Part print with two shaded views. Sizes in mm from the minimum x, y, z corner. A direction names the side the tool comes from. Coordinates: 2 decimals unless noted, no trailing zeros. Order: outer loops, then holes, each group sorted by start corner. A loop starts at its lowest first (then second) coordinate and runs counter-clockwise, first axis right, second up.
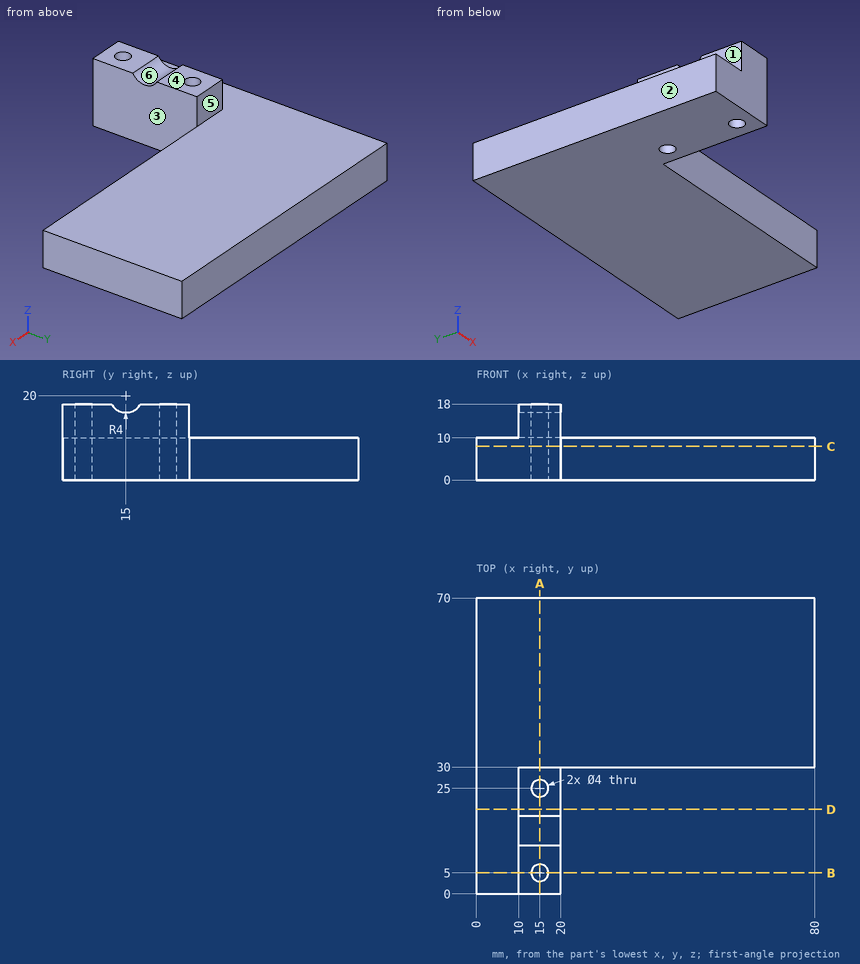
Q1. Cut at A-A on x = 15. Write the cut outline in (y, z).
Results list:
outline: (0, 0) - (3, 0) - (3, 18) - (0, 18) - close; (7, 0) - (23, 0) - (23, 18) - (18.46, 18) arc R4 cw to (11.54, 18) - (7, 18) - close; (27, 0) - (70, 0) - (70, 10) - (30, 10) - (30, 18) - (27, 18) - close
Q2. Wall check: line 1 along Y through (x, z) = (15, 9.25); line 2 along X through (y, z) = (25, 6.25); line 3 along X through (y, z) = (25, 11.25). Give the ranges that are in metal, low to high.
Results list:
line 1: y = 0 to 3, 7 to 23, 27 to 70
line 2: x = 0 to 13, 17 to 20
line 3: x = 10 to 13, 17 to 20
Q3. Pin check, flat tips, straight feed: pin 1 Ø1 at (x, y) = (68.5, 58.5) entering from +Z; pin 2 Ø5 at (x, z) = (37.5, 14.5) entering from +Y; pin 3 Ø8 at (x, z) = (35.5, 4) entering from -Y; pin 4 Ø2.5 at (y, z) = (17.5, 13.5) entering from -X. Stop position of each tip, or through.
Results list:
pin 1: stops at z = 10
pin 2: passes through
pin 3: stops at y = 30
pin 4: stops at x = 10
Q4. Cut at B-B on y = 5. Write the cut outline in (x, z).
Results list:
outline: (0, 0) - (13, 0) - (13, 18) - (10, 18) - (10, 10) - (0, 10) - close; (17, 0) - (20, 0) - (20, 18) - (17, 18) - close
Q5. Cut at C-C on z = 8. Write the cut outline in (x, y), and give its area (3 significant figures).
Results list:
outline: (0, 0) - (20, 0) - (20, 30) - (80, 30) - (80, 70) - (0, 70) - close; hole circle Ø4 at (15, 5); hole circle Ø4 at (15, 25)
area: 3,770 mm2
Q6. Cut at D-D on y = 20. Write the cut outline in (x, z).
Results list:
outline: (0, 0) - (20, 0) - (20, 18) - (10, 18) - (10, 10) - (0, 10) - close
Q7. Mould opens along Y. For the marked faces 4, 5 and 6 say: pulls with the +Y half, pulls with the -Y half, needs draft (parallel to the pull), parting line crosses it, or undercut.
Results list:
face 4: needs draft
face 5: pulls with the +Y half
face 6: undercut
Q8. Which spindle directions (+Z, -Z, +X, -X, +Y, -Y) get a long thin tool onto all of the face, cutting with end or side? Do the marked faces 1, 2 and 3. Say none if no direction does.
Results list:
face 1: +Z, -X, +Y, -Y
face 2: +Z, -Z, -X, +Y, -Y
face 3: +Z, -Z, +X, -Y
